from build123d import *

# Parameters (mm, degrees)
BOSS_EXTRUDE1_DEPTH = 10
SKETCH3_R           = 3.96875
CUT_EXTRUDE1_DEPTH  = 662.513416342
SKETCH4_R           = 25
CUT_EXTRUDE2_DEPTH  = 662.513416342
CIRPATTERN2_COUNT   = 6


with BuildPart() as part:
    # Sketch1 → Boss-Extrude1 (new body)
    with BuildSketch(Plane(origin=(0, 0, 0), x_dir=(1, 0, 0), z_dir=(0, 1, 0))):
        Polygon((500, 0), (250, 433.012701892), (-250, 433.012701892), (-500, 0), (-250, -433.012701892), (250, -433.012701892), align=None)
    extrude(amount=BOSS_EXTRUDE1_DEPTH)

    # Sketch3 → Cut-Extrude1 (cut, through all)
    with BuildSketch(Plane.XZ):
        with Locations(Location((187.522727339, 295.878891325, 0), (0, 0, 270))):
            Circle(SKETCH3_R)
        with Locations(Location((162.477272661, 310.338891325, 0), (0, 0, 270))):
            Circle(SKETCH3_R)
    cut_extrude1 = extrude(amount=-CUT_EXTRUDE1_DEPTH, mode=Mode.SUBTRACT)

    # Sketch4 → Cut-Extrude2 (cut, through all)
    with BuildSketch(Plane.XZ):
        with Locations(Location((0, 0, 0), (0, 0, 270))):
            Circle(SKETCH4_R)
    extrude(amount=-CUT_EXTRUDE2_DEPTH, mode=Mode.SUBTRACT)

    # CirPattern2: Cut-Extrude1 ×6 about axis
    cirpattern2_axis = Axis((0, 0, 0), (0, 1, 0))
    for i in range(1, CIRPATTERN2_COUNT):
        add(cut_extrude1.rotate(cirpattern2_axis, i * 360 / CIRPATTERN2_COUNT), mode=Mode.SUBTRACT)


solid = part.part
For this review, take the finished solid that the model builds, in its own axes (mm). Give positions to 0.01 mm unless a question says otherwise; leave off trailing zeros. Loops run counter-clockwise (first coordinate to the right, second up) from the corner with the lowest first, then second, coordinate; pieces in that order, holes last.
Item 1: Take a section at C-C, the plane z = -254. State the section outline as (x, y) points, and give its area (3 significant figures).
Item 2: For line 1 along X through (y, z) = (6, -14.46); line 2 along Z through (x, y) = (188.5, 6); line 3 along Z through (x, y) = (-350, 5), list the stretches that pass through material, from the lowest coordinate up.
Item 3: Insertion check: pin 1 (12.5 mm diameter, centred on x = -162.48, z = -310.34, fed in from -Y); pin 2 (7 mm diameter, centred on x = -350, z = 14.46, fed in from +Y); pin 3 (3 mm diameter, centred on y = 3.5, z = 234, fed in from -X); pin 4 (3 mm diameter, centred on x = 376, y = 3.5, fed in from -Z). Each pin has a flat end and moves straight along its axis. Give the tip position at first contact, or say it passes through.
Item 4: Draft analysis for pull direction Z (two halves, no side actions). For faces 1 (the flat face through (104, 10, -6)), 2 (the cylindrical face through (7.509, 4.93, -23.846)), 3 (the flat face through (-373.25, 4.93, -219.54)), state which applies: +Z half, -Z half, draft (parallel to the pull), parting line (faces both ways), or undercut.
Item 5: Take a section at B-B, the plane y = 5.5. Give the number of separate pieces and of enclosed holes in the cut face, and give its area (3 significant figures).
Item 6: Take a section at D-D, the plane x = 319.5. State the section outline as (y, z) points, and give its area (3 significant figures).
Item 7: Take a section at A-A, the plane x = 0. State the section outline as (y, z) points, and give its area (3 significant figures).
Calculated:
1. outline: (-353.35, 0) - (353.35, 0) - (353.35, 10) - (-353.35, 10) - close
1. area: 7,070 mm2
2. line 1: x = -491.65 to -353.97, -346.03 to -20.39, 20.39 to 346.03, 353.97 to 491.65
2. line 2: z = -433.01 to -299.73, -292.03 to 292.03, 299.73 to 433.01
2. line 3: z = -259.81 to -18.43, -10.49 to 10.49, 18.43 to 259.81
3. pin 1: stops at y = 0
3. pin 2: passes through
3. pin 3: stops at x = -365.77
3. pin 4: stops at z = -217.37
4. face 1: draft
4. face 2: undercut
4. face 3: -Z half
5. separate pieces: 1
5. enclosed holes: 13
5. area: 647,000 mm2
6. outline: (0, -312.64) - (10, -312.64) - (10, 312.64) - (0, 312.64) - close
6. area: 6,250 mm2
7. outline: (0, -433.01) - (10, -433.01) - (10, -25) - (0, -25) - close; (0, 25) - (10, 25) - (10, 433.01) - (0, 433.01) - close
7. area: 8,160 mm2
